Model file for the job. Use its own axes, mm. A direction names the side the tool comes from. Give positions to 0.01 mm unless a question says otherwise; leave off trailing zeros. Loops run counter-clockwise (first coordinate to the right, second up) from the corner with the lowest first, then second, coordinate; pieces in that order, holes last. Notation, with made-up numbers: M 87,59 L 129,59 A21 cw 129,82 Z; hole C -38.5,60 d8. An arc over 180 degrees is marked long. Use CSV: the item, a comma, the result in double quotes. Start each with the question number.
(1) Flat gauge pins, fed straight in: P1, Ø1.6, axis at y = -79, z = 1.5, coming from the -X side; P2, Ø4, axis at x = -45, y = 111, coming from the -Z side; P3, Ø1, axis at y = -70, z = 2.5, coming from the -X side. Where does each tip first touch, or does it go through?
(2) Two-plate mould, pull along X, no slides. Class faces 1 (the face through (-231.141, -155.954, 1.565)), 2 (the face through (232.47, -155.47, 1.57)), 3 (the face through (4, 2, 3.175)): pulls with the +X half, pulls with the -X half, needs draft (parallel to the pull), parting line crosses it, or undercut.
(3) Tool access for faces 4 (the face through (-197.74, 68.56, 1.61)), 5 (the face through (-232.47, 155.47, 1.57)): list every direction of +Z, -Z, +X, -X, +Y, -Y with a clear straight run to the whole face (end or side of a thin tool).
(4) Wall check: line 1 along X through (y, z) = (-30.5, 1.7); line 2 along Y through (x, z) = (57.5, 1.55); line 3 along X through (y, z) = (-102, 0.9). Give the ranges that are in metal, low to high. Write a range as from..to.
(5) Slice it at A-A on y = 9. List the corners of the cut face in (x, z) (3 decimals).
(6) Slice it at B-B on y = -148.5. List the corners of the cut face in (x, z) (3 decimals), and give its area (3 significant figures).
(7) Slice it at C-C on z = 1.5. State how many separate pieces and enclosed holes the cut face has, and give its area (3 significant figures).
```python
from build123d import *

# Parameters (mm, degrees)
BOSS_EXTRUDE1_DEPTH = 3.175
FILLET3_R           = 25.4
CUT_EXTRUDE3_DEPTH  = 4.175


with BuildPart() as part:
    # Sketch1 → Boss-Extrude1 (new body)
    with BuildSketch(Plane.XY):
        Polygon((-279.4, 138.38935405), (-184.214073546, 173.034198), (184.214073546, 173.034198), (279.4, 138.38935405), (279.4, -138.38935405), (184.214073546, -173.034198), (-184.214073546, -173.034198), (-279.4, -138.38935405), (-279.4, -76.2), (-190.5, -76.2), (-190.5, 76.2), (-279.4, 76.2), align=None)
    extrude(amount=BOSS_EXTRUDE1_DEPTH)

    # Fillet3
    fillet3_edges = [part.edges().sort_by_distance(p)[0] for p in [
        (-279.4, -76.2, 1.5875),
        (-190.5, -76.2, 1.5875),
        (-190.5, 76.2, 1.5875),
        (-279.4, 76.2, 1.5875),
    ]]
    fillet(fillet3_edges, radius=FILLET3_R)

    # Sketch4 → Cut-Extrude3 (cut, through all)
    with BuildSketch(Plane.XY.offset(3.175)):
        with BuildLine():
            Line((-254, 98.6282), (-31.75, 98.6282))
            ThreePointArc((-31.75, 98.6282), (-28.3718, 95.25), (-31.75, 91.8718))
            Line((-31.75, 91.8718), (-254, 91.8718))
            ThreePointArc((-254, 91.8718), (-257.3782, 95.25), (-254, 98.6282))
        make_face()
        with BuildLine():
            Line((-201.660555159, 117.6782), (-31.75, 117.6782))
            ThreePointArc((-31.75, 117.6782), (-28.3718, 114.3), (-31.75, 110.9218))
            Line((-31.75, 110.9218), (-201.660555159, 110.9218))
            ThreePointArc((-201.660555159, 110.9218), (-205.038755159, 114.3), (-201.660555159, 117.6782))
        make_face()
        with BuildLine():
            Line((-149.321110319, 136.7282), (-31.75, 136.7282))
            ThreePointArc((-31.75, 136.7282), (-28.3718, 133.35), (-31.75, 129.9718))
            Line((-31.75, 129.9718), (-149.321110319, 129.9718))
            ThreePointArc((-149.321110319, 129.9718), (-152.699310319, 133.35), (-149.321110319, 136.7282))
        make_face()
        with BuildLine():
            Line((-161.7218, 69.85), (-161.7218, -69.85))
            ThreePointArc((-161.7218, -69.85), (-165.1, -73.2282), (-168.4782, -69.85))
            Line((-168.4782, -69.85), (-168.4782, 69.85))
            ThreePointArc((-168.4782, 69.85), (-165.1, 73.2282), (-161.7218, 69.85))
        make_face()
        with BuildLine():
            Line((-110.9218, 69.85), (-110.9218, -69.85))
            ThreePointArc((-110.9218, -69.85), (-114.3, -73.2282), (-117.6782, -69.85))
            Line((-117.6782, -69.85), (-117.6782, 69.85))
            ThreePointArc((-117.6782, 69.85), (-114.3, 73.2282), (-110.9218, 69.85))
        make_face()
        with BuildLine():
            Line((31.75, 114.3), (50.8, 114.3))
            ThreePointArc((50.8, 114.3), (55.290128061, 112.440128061), (57.15, 107.95))
            Line((57.15, 107.95), (57.15, 57.15))
            ThreePointArc((57.15, 57.15), (55.290128061, 52.659871939), (50.8, 50.8))
            Line((50.8, 50.8), (31.75, 50.8))
            ThreePointArc((31.75, 50.8), (27.259871939, 52.659871939), (25.4, 57.15))
            Line((25.4, 57.15), (25.4, 107.95))
            ThreePointArc((25.4, 107.95), (27.259871939, 112.440128061), (31.75, 114.3))
        make_face()
        with BuildLine():
            Line((3.3782, 160.334198), (3.3782, 44.45))
            ThreePointArc((3.3782, 44.45), (0, 41.0718), (-3.3782, 44.45))
            Line((-3.3782, 44.45), (-3.3782, 160.334198))
            ThreePointArc((-3.3782, 160.334198), (0, 163.712398), (3.3782, 160.334198))
        make_face()
        with BuildLine():
            Line((-88.9, 28.7782), (254, 28.7782))
            ThreePointArc((254, 28.7782), (257.3782, 25.4), (254, 22.0218))
            Line((254, 22.0218), (-88.9, 22.0218))
            ThreePointArc((-88.9, 22.0218), (-92.2782, 25.4), (-88.9, 28.7782))
        make_face()
        with BuildLine():
            Line((79.1718, 44.45), (79.1718, 160.334198))
            ThreePointArc((79.1718, 160.334198), (82.55, 163.712398), (85.9282, 160.334198))
            Line((85.9282, 160.334198), (85.9282, 44.45))
            ThreePointArc((85.9282, 44.45), (82.55, 41.0718), (79.1718, 44.45))
        make_face()
        with BuildLine():
            Line((111.3282, 160.334198), (111.3282, 44.45))
            ThreePointArc((111.3282, 44.45), (107.95, 41.0718), (104.5718, 44.45))
            Line((104.5718, 44.45), (104.5718, 160.334198))
            ThreePointArc((104.5718, 160.334198), (107.95, 163.712398), (111.3282, 160.334198))
        make_face()
        with BuildLine():
            Line((133.35, 124.0282), (184.214073546, 124.0282))
            ThreePointArc((184.214073546, 124.0282), (187.592273546, 120.65), (184.214073546, 117.2718))
            Line((184.214073546, 117.2718), (133.35, 117.2718))
            ThreePointArc((133.35, 117.2718), (129.9718, 120.65), (133.35, 124.0282))
        make_face()
        with BuildLine():
            Line((133.35, 98.6282), (254, 98.6282))
            ThreePointArc((254, 98.6282), (257.3782, 95.25), (254, 91.8718))
            Line((254, 91.8718), (133.35, 91.8718))
            ThreePointArc((133.35, 91.8718), (129.9718, 95.25), (133.35, 98.6282))
        make_face()
        with BuildLine():
            Line((133.35, 73.2282), (266.7, 73.2282))
            ThreePointArc((266.7, 73.2282), (270.0782, 69.85), (266.7, 66.4718))
            Line((266.7, 66.4718), (133.35, 66.4718))
            ThreePointArc((133.35, 66.4718), (129.9718, 69.85), (133.35, 73.2282))
        make_face()
        with BuildLine():
            Line((133.35, 47.8282), (266.7, 47.8282))
            ThreePointArc((266.7, 47.8282), (270.0782, 44.45), (266.7, 41.0718))
            Line((266.7, 41.0718), (133.35, 41.0718))
            ThreePointArc((133.35, 41.0718), (129.9718, 44.45), (133.35, 47.8282))
        make_face()
        with BuildLine():
            Line((-254, -98.6282), (-31.75, -98.6282))
            ThreePointArc((-31.75, -98.6282), (-28.3718, -95.25), (-31.75, -91.8718))
            Line((-31.75, -91.8718), (-254, -91.8718))
            ThreePointArc((-254, -91.8718), (-257.3782, -95.25), (-254, -98.6282))
        make_face()
        with BuildLine():
            Line((-201.660555159, -117.6782), (-31.75, -117.6782))
            ThreePointArc((-31.75, -117.6782), (-28.3718, -114.3), (-31.75, -110.9218))
            Line((-31.75, -110.9218), (-201.660555159, -110.9218))
            ThreePointArc((-201.660555159, -110.9218), (-205.038755159, -114.3), (-201.660555159, -117.6782))
        make_face()
        with BuildLine():
            Line((-149.321110319, -136.7282), (-31.75, -136.7282))
            ThreePointArc((-31.75, -136.7282), (-28.3718, -133.35), (-31.75, -129.9718))
            Line((-31.75, -129.9718), (-149.321110319, -129.9718))
            ThreePointArc((-149.321110319, -129.9718), (-152.699310319, -133.35), (-149.321110319, -136.7282))
        make_face()
        with BuildLine():
            Line((3.3782, -160.334198), (3.3782, -44.45))
            ThreePointArc((3.3782, -44.45), (0, -41.0718), (-3.3782, -44.45))
            Line((-3.3782, -44.45), (-3.3782, -160.334198))
            ThreePointArc((-3.3782, -160.334198), (0, -163.712398), (3.3782, -160.334198))
        make_face()
        with BuildLine():
            Line((-88.9, -28.7782), (254, -28.7782))
            ThreePointArc((254, -28.7782), (257.3782, -25.4), (254, -22.0218))
            Line((254, -22.0218), (-88.9, -22.0218))
            ThreePointArc((-88.9, -22.0218), (-92.2782, -25.4), (-88.9, -28.7782))
        make_face()
        with BuildLine():
            Line((79.1718, -44.45), (79.1718, -160.334198))
            ThreePointArc((79.1718, -160.334198), (82.55, -163.712398), (85.9282, -160.334198))
            Line((85.9282, -160.334198), (85.9282, -44.45))
            ThreePointArc((85.9282, -44.45), (82.55, -41.0718), (79.1718, -44.45))
        make_face()
        with BuildLine():
            Line((111.3282, -160.334198), (111.3282, -44.45))
            ThreePointArc((111.3282, -44.45), (107.95, -41.0718), (104.5718, -44.45))
            Line((104.5718, -44.45), (104.5718, -160.334198))
            ThreePointArc((104.5718, -160.334198), (107.95, -163.712398), (111.3282, -160.334198))
        make_face()
        with BuildLine():
            Line((133.35, -124.0282), (184.214073546, -124.0282))
            ThreePointArc((184.214073546, -124.0282), (187.592273546, -120.65), (184.214073546, -117.2718))
            Line((184.214073546, -117.2718), (133.35, -117.2718))
            ThreePointArc((133.35, -117.2718), (129.9718, -120.65), (133.35, -124.0282))
        make_face()
        with BuildLine():
            Line((133.35, -98.6282), (254, -98.6282))
            ThreePointArc((254, -98.6282), (257.3782, -95.25), (254, -91.8718))
            Line((254, -91.8718), (133.35, -91.8718))
            ThreePointArc((133.35, -91.8718), (129.9718, -95.25), (133.35, -98.6282))
        make_face()
        with BuildLine():
            Line((133.35, -73.2282), (266.7, -73.2282))
            ThreePointArc((266.7, -73.2282), (270.0782, -69.85), (266.7, -66.4718))
            Line((266.7, -66.4718), (133.35, -66.4718))
            ThreePointArc((133.35, -66.4718), (129.9718, -69.85), (133.35, -73.2282))
        make_face()
        with BuildLine():
            Line((133.35, -47.8282), (266.7, -47.8282))
            ThreePointArc((266.7, -47.8282), (270.0782, -44.45), (266.7, -41.0718))
            Line((266.7, -41.0718), (133.35, -41.0718))
            ThreePointArc((133.35, -41.0718), (129.9718, -44.45), (133.35, -47.8282))
        make_face()
        with BuildLine():
            Line((57.15, -107.95), (57.15, -57.15))
            ThreePointArc((57.15, -57.15), (55.290128061, -52.659871939), (50.8, -50.8))
            Line((50.8, -50.8), (31.75, -50.8))
            ThreePointArc((31.75, -50.8), (27.259871939, -52.659871939), (25.4, -57.15))
            Line((25.4, -57.15), (25.4, -107.95))
            ThreePointArc((25.4, -107.95), (27.259871939, -112.440128061), (31.75, -114.3))
            Line((31.75, -114.3), (50.8, -114.3))
            ThreePointArc((50.8, -114.3), (55.290128061, -112.440128061), (57.15, -107.95))
        make_face()
        with BuildLine():
            Line((25.4, 3.3782), (215.9, 3.3782))
            ThreePointArc((215.9, 3.3782), (219.2782, 0), (215.9, -3.3782))
            Line((215.9, -3.3782), (25.4, -3.3782))
            ThreePointArc((25.4, -3.3782), (22.0218, 0), (25.4, 3.3782))
        make_face()
    extrude(amount=-CUT_EXTRUDE3_DEPTH, mode=Mode.SUBTRACT)


solid = part.part
```
Reply:
1,P1,"stops at x = -267.04"
1,P2,"stops at z = 0"
1,P3,"stops at x = -199.87"
2,face 1,"pulls with the -X half"
2,face 2,"pulls with the +X half"
2,face 3,"needs draft"
3,face 4,"+Z, -Z, -X"
3,face 5,"+Z, -Z, -X, +Y"
4,line 1,"x = -190.5..-168.48, -161.72..-117.68, -110.92..279.4"
4,line 2,"y = -173.03..-28.78, -22.02..-3.38, 3.38..22.02, 28.78..173.03"
4,line 3,"x = -279.4..-3.38, 3.38..25.4, 57.15..79.17, 85.93..104.57, 111.33..279.4"
5,outline,"M -190.5,0 L -168.478,0 L -168.478,3.175 L -190.5,3.175 Z; M -161.722,0 L -117.678,0 L -117.678,3.175 L -161.722,3.175 Z; M -110.922,0 L 279.4,0 L 279.4,3.175 L -110.922,3.175 Z"
6,outline,"M -251.621,0 L -3.378,0 L -3.378,3.175 L -251.621,3.175 Z; M 3.378,0 L 79.172,0 L 79.172,3.175 L 3.378,3.175 Z; M 85.928,0 L 104.572,0 L 104.572,3.175 L 85.928,3.175 Z; M 111.328,0 L 251.621,0 L 251.621,3.175 L 111.328,3.175 Z"
6,area,"1,530 mm^2"
7,separate pieces,"1"
7,enclosed holes,"27"
7,area,"143,000 mm^2"
